Autodesk Fusion 360 part; units mm, degrees
sketch "Sketch1" plane through (0, 0, 0) normal (0, 0, 1) x (1, 0, 0)
  line L0 (0, 0) -> (0, 98) construction
  line L1 (0, 98) -> (20, 118) construction
  line L2 (20, 118) -> (30, 118) construction
  line L3 (9, 0) -> (9, 94.2721)
  line L4 (9, 94.2721) -> (23.7279, 109)
  line L5 (23.7279, 109) -> (30, 109)
  line L6 (-3, 0) -> (-3, 99.2426)
  line L7 (-3, 99.2426) -> (18.7574, 121)
  line L8 (18.7574, 121) -> (30, 121)
  line L9 (0, 0) -> (9, 0) construction
  line L10 (0, 0) -> (-3, 0) construction
  line L11 (30, 118) -> (30, 109)
  line L12 (30, 118) -> (30, 121)
  line L13 (0, -3) -> (9, -3)
  line L14 (0, -3) -> (-3, -3)
  line L15 (9, -3) -> (9, 0)
  line L16 (-3, -3) -> (-3, 0)
  dimension "d7" = 98
  dimension "d8" = 135
  dimension "d9" = 118
  dimension "d10" = 10
  dimension "d11" = 9
  dimension "d12" = -3
  dimension "d13" = 3
extrude "Extrude1" add sketch "Sketch1" along normal blind 37.22
shell "Shell1" thickness 3 removed faces 4 at (30, 119, 12.4067) at (25.8186, 109, 12.4067) at (13.9093, 99.1814, 24.8133) at (9, 31.424, 12.4067)
sketch "Sketch2" plane through (-3, 0, 0) normal (-1, 0, 0) x (0, -1, 0)
  line L0 (-99.2426, 0) -> (3, 0)
  line L1 (3, 0) -> (3, 37.22)
  line L2 (3, 37.22) -> (-99.2426, 37.22)
  line L3 (-99.2426, 37.22) -> (-99.2426, 0)
  line L4 (0, 3) -> (-98, 3) construction
  line L5 (-98, 3) -> (-98, 34.22) construction
  line L6 (-98, 34.22) -> (0, 34.22) construction
  line L7 (0, 34.22) -> (0, 3) construction
  circle A0 centre (-5, 29.22) radius 2
  circle A1 centre (-93, 8) radius 1.3
  circle A2 centre (-93, 8) radius 2
  circle A3 centre (-5, 29.22) radius 1.3
  dimension "d21" = 3
  dimension "d22" = 3
  dimension "d23" = 3
  dimension "d24" = 98
  dimension "d25" = 2.6
  dimension "d26" = 4
  dimension "d27" = 5
  dimension "d28" = 5
  dimension "d29" = 5
  dimension "d30" = 5
  dimension "d31" = 2.6
  dimension "d32" = 4
extrude "Extrude2" cut sketch "Sketch2" against normal through all contours A1 | A3
extrude "Extrude3" cut sketch "Sketch2" against normal blind 2 contours A0 | A2
fillet "Fillet3" radius 1.5 10 edges at (-3, -3, 18.61) (-3, 48.1213, 37.22) (-3, 48.1213, 0) (-3, 99.2426, 18.61) (7.8787, 110.1213, 37.22) (7.8787, 110.1213, 0) (18.7574, 121, 18.61) (24.3787, 121, 37.22) (24.3787, 121, 0) (30, 121, 18.61)
The listing builds one solid part. Answer for the finished solid, in the listing's coordinates (mm). A direction names the side the tool comes from. Round coordinates to 2 decimals unless told otherwise and drop trailing zeros. Loops run counter-clockwise (first coordinate to the right, second up) from the corner with the lowest first, then second, coordinate; pieces in that order, holes last. Notation, with made-up numbers: (85, 72.5) - (113, 72.5) arc R16 cw to (113, 97.5) - close; hole circle Ø1 at (-15.75, -26.75). An arc over 180 degrees is marked (long way). Return JSON: item names as keys, results as strings. Group by question number.
1. The part is cut by section D-D on x = 25. Determine the outline of the cut face in (y, z).
2. Consider probe 1 along Z at (x, y) = (1, 93); probe 2 along Z at (x, y) = (3, 5); probe 3 along X at (y, z) = (86.5, 10.5). Determine where each line is inside the solid, lowest interval first.
3. Which of the six approach directions +Z, -Z, +X, -X, +Y, -Y give full straight-line access (tool end or side, diameter ignored) to faces 1 (the flat face through (27, 109, 18)), 2 (the cylindrical face through (-2.014, 91.092, 8.601)), 3 (the cylindrical face through (8.327, 109.965, 36.769))?
4. The part is cut by section C-C on z = 13. Determine the outline of the cut face in (x, y).
5. The mould has two halves that part along Z. Classify faces 4 (the cylindrical face through (3.93, 5.17, 30.51)), 5 (the flat face through (7, 59, 37.22)), 6 (the flat face through (9, 45, 18)): pulls with the +Z half, pulls with the -Z half, needs draft (parallel to the pull), parting line crosses it, or undercut.
6. The part is cut by section A-A on y = 93. Determine the outline of the cut face in (x, z).
7. Each of these flat-tipped pins is pushed along its axis until it touches: P1, Ø1.2, axis at y = 92.5, z = 7, coming from the -X side; P2, Ø3, axis at y = 18.5, z = 25.5, coming from the +X side; P3, Ø3, axis at x = 26, z = 26, coming from the -Y side. Where does it stop, or does it pass through?
8. The part is cut by section B-B on z = 29.22. Determine the outline of the cut face in (x, y).
Resolved:
{
 "1": {"outline": "(109, 0) - (119.5, 0) arc R1.5 ccw to (121, 1.5) - (121, 35.72) arc R1.5 ccw to (119.5, 37.22) - (109, 37.22) - close"},
 "2": {"probe 1": "z = 0 to 6.7, 9.3 to 37.22", "probe 2": "z = 0 to 27.92, 30.52 to 37.22", "probe 3": "x = -3 to 9"},
 "3": {"face 1": "+Z, -Z, +X, -Y", "face 2": "-X", "face 3": "+Z, -X, +Y"},
 "4": {"outline": "(-3, -1.5) arc R1.5 ccw to (-1.5, -3) - (9, -3) - (9, 94.27) - (23.73, 109) - (30, 109) - (30, 119.5) arc R1.5 ccw to (28.5, 121) - (19.38, 121) arc R1.5 ccw to (18.32, 120.56) - (-2.56, 99.68) arc R1.5 ccw to (-3, 98.62) - close"},
 "5": {"face 4": "undercut", "face 5": "pulls with the +Z half", "face 6": "needs draft"},
 "6": {"outline": "(-3, 1.5) arc R1.5 ccw to (-1.5, 0) - (9, 0) - (9, 6.7) - (-1, 6.7) - (-1, 6) - (-3, 6) - close; (-3, 10) - (-1, 10) - (-1, 9.3) - (9, 9.3) - (9, 37.22) - (-1.5, 37.22) arc R1.5 ccw to (-3, 35.72) - close"},
 "7": {"P1": "stops at x = -1", "P2": "stops at x = 9", "P3": "stops at y = 109"},
 "8": {"outline": "(-3, -1.5) arc R1.5 ccw to (-1.5, -3) - (9, -3) - (9, 3.7) - (-1, 3.7) - (-1, 3) - (-3, 3) - close; (-3, 7) - (-1, 7) - (-1, 6.3) - (9, 6.3) - (9, 94.27) - (23.73, 109) - (30, 109) - (30, 119.5) arc R1.5 ccw to (28.5, 121) - (19.38, 121) arc R1.5 ccw to (18.32, 120.56) - (-2.56, 99.68) arc R1.5 ccw to (-3, 98.62) - close"}
}
